Design review of the part built by this model. Coordinates are the model's own, in mm. A direction names the side the tool comes from. Coordinates: 2 decimals unless noted, no trailing zeros. Write each loop counter-clockwise with the first axis right and the second up, starting at its lowest first coordinate (ties: lowest second). Pieces come first, ordered by that corner, then holes.
Q1. Clearance check with flat-ended pins moving along their axes: pin 1 Ø2.5 at (y, z) = (-44.5, 3.5) entering from -X; pin 2 Ø0.9 at (y, z) = (10, 1.5) entering from +X; pin 3 Ø0.8 at (x, z) = (35.5, 2.5) entering from -Y. State where each tip first meets the part, or that it passes through.
Q2. Add section D-D, the plane y = -39. Give the boundary of the cut face in (x, z), plus the area to 3 significant figures.
Q3. To check wall thickness, follow probe 1 along Y at (x, z) = (1, 3.3); probe 2 along Y at (x, z) = (9, 0.4); probe 3 along X at (y, z) = (13, 0.85). State the ranges of each line that lie inside material, in increasing order.
Q4. Add section C-C, the plane z = 1.2. Give the number of separate pieces and of enclosed holes in the cut face, plus the area to 3 significant figures.
Q5. The part is to be moulded in two halves that separate along X. For faces 6 (the face through (-51, 10, 2)), 7 (the face through (23, 29.796, 2)), 8 (the face through (-5, 35.796, 2)), say which applies: +X half, -X half, draft (parallel to the pull), parting line (faces both ways), or undercut.
Q6. Machinability: for faces 1 (the face through (24, 34.796, 2)), 2 (the face through (-6, 1, 5)), 3 (the face through (-16, -42, 2)), 4 (the face through (42, 15, 2)), 5 (the face through (-41.43, -17.01, 2.46)), which of the approach directions +Z, -Z, +X, -X, +Y, -Y give a long, thin tool a straight path to every point of the face, cutting with its end or side? Answer none if there is none.
Q7. Add section B-B, the plane y = -19.5. Give the boundary of the cut face in (x, z) (3 decimals).
Q8. Add section A-A, the plane x = -20.5. Give the boundary of the cut face in (y, z).
from build123d import *

# Parameters (mm, degrees)
BOSS_EXTRU_1_DEPTH = 5


with BuildPart() as part:
    # Esquisse1 → Boss.-Extru.1 (new body)
    with BuildSketch(Plane.XY):
        Polygon((-32, -29.022213998), (-32, -30.022213998), (-16, -30.022213998), (-16, -55.022213998), (6, -55.022213998), (6, -30.022213998), (22, -30.022213998), (22, -29.022213998), (25, -29.022213998), (25, -30.022213998), (32, -30.022213998), (42, -12.701705922), (42, -5.701705922), (41, -5.701705922), (41, -2.701705922), (42, -2.701705922), (42, 8.475208614), (41, 8.475208614), (41, 11.475208614), (42, 11.475208614), (42, 18.475208614), (32, 35.79571669), (25, 35.79571669), (25, 34.79571669), (22, 34.79571669), (22, 35.79571669), (-32, 35.79571669), (-32, 34.79571669), (-35, 34.79571669), (-35, 35.79571669), (-42, 35.79571669), (-52, 18.475208614), (-52, 11.475208614), (-51, 11.475208614), (-51, 8.475208614), (-52, 8.475208614), (-52, -2.701705922), (-51, -2.701705922), (-51, -5.701705922), (-52, -5.701705922), (-52, -12.701705922), (-42, -30.022213998), (-35, -30.022213998), (-35, -29.022213998), align=None)
        Polygon((-46, -2.701705922), (-45, -2.701705922), (35, -2.701705922), (36, -2.701705922), (36, -5.701705922), (35, -5.701705922), (35, -10.826061575), (27.958548116, -23.022213998), (25, -23.022213998), (25, -24.022213998), (22, -24.022213998), (22, -23.022213998), (-32, -23.022213998), (-32, -24.022213998), (-35, -24.022213998), (-35, -23.022213998), (-37.958548116, -23.022213998), (-45, -10.826061575), (-45, -5.701705922), (-46, -5.701705922), align=None, mode=Mode.SUBTRACT)
        Polygon((-45, 2.886751346), (-45, 8.475208614), (-46, 8.475208614), (-46, 11.475208614), (-45, 11.475208614), (-45, 14.177208614), (-41.5, 14.177208614), (-41.5, 2.886751346), align=None, mode=Mode.SUBTRACT)
        Polygon((-32, 29.79571669), (-32, 28.79571669), (22, 28.79571669), (22, 29.79571669), (25, 29.79571669), (25, 28.79571669), (27.958548116, 28.79571669), (27.958548116, 19.842608257), (-37.958548116, 19.842608257), (-37.958548116, 28.79571669), (-35, 28.79571669), (-35, 29.79571669), align=None, mode=Mode.SUBTRACT)
        Polygon((35, 8.475208614), (35, 2.886751346), (31.5, 2.886751346), (31.5, 14.177208614), (35, 14.177208614), (35, 11.475208614), (36, 11.475208614), (36, 8.475208614), align=None, mode=Mode.SUBTRACT)
    extrude(amount=BOSS_EXTRU_1_DEPTH)


solid = part.part
Here are the results:
1. pin 1: stops at x = -16
1. pin 2: stops at x = 41
1. pin 3: stops at y = -24.65
2. outline: (-16, 0) - (6, 0) - (6, 5) - (-16, 5) - close
2. area: 110 mm2
3. probe 1: y = -55.02 to -23.02, -2.7 to 19.84, 28.8 to 35.8
3. probe 2: y = -30.02 to -23.02, -2.7 to 19.84, 28.8 to 35.8
3. probe 3: x = -52 to -45, -41.5 to 31.5, 35 to 42
4. separate pieces: 1
4. enclosed holes: 4
4. area: 4,130 mm2
5. face 6: -X half
5. face 7: undercut
5. face 8: draft
6. face 1: +Z, -Z, +Y
6. face 2: +Z, +X, -X, +Y, -Y
6. face 3: +Z, -Z, -X, -Y
6. face 4: +Z, -Z, +X, +Y, -Y
6. face 5: +Z, -Z
7. outline: (-48.075, 0) - (-39.992, 0) - (-39.992, 5) - (-48.075, 5) - close; (29.992, 0) - (38.075, 0) - (38.075, 5) - (29.992, 5) - close
8. outline: (-30.02, 0) - (-23.02, 0) - (-23.02, 5) - (-30.02, 5) - close; (-2.7, 0) - (19.84, 0) - (19.84, 5) - (-2.7, 5) - close; (28.8, 0) - (35.8, 0) - (35.8, 5) - (28.8, 5) - close
